Design review of the part built by this model. Coordinates are the model's own, in mm. A direction names the side the tool comes from. Coordinates: 2 decimals unless noted, no trailing zeros. Loops run counter-clockwise (first coordinate to the right, second up) from the corner with the lowest first, then second, coordinate; pieces in that order, holes last.
from build123d import *

# Parameters (mm, degrees)
SERVO_SHELF_START                        = -36.480025
SKETCH1_W                                = 48
SKETCH1_H                                = 38
SKETCH1_W_2                              = 13
SKETCH1_H_2                              = 24.35
SERVO_SHELF_DEPTH                        = 3
OUTBOARD_RISER_START                     = -34.480025
SKETCH2_W                                = 6
SKETCH2_H                                = 14
OUTBOARD_RISER_DEPTH                     = 33.480025
PLATE_ATTACHMENT_FOOT_START              = -2
SKETCH3_W                                = 20
SKETCH3_H                                = 14
PLATE_ATTACHMENT_FOOT_DEPTH              = 2
SKETCH4_R                                = 1.45
SERVO_PAD_D2P9_DEPTH                     = 2.01
SKETCH5_R                                = 2.6
SERVO_PAD_CSK_D5P2_90DEG_DEPTH           = 1.15
SERVO_PAD_CSK_D5P2_90DEG_DRAFT           = -45
SERVO_PAD_CSK_D5P2_90DEG_PROFILE_2_DEPTH = 1.15
SERVO_PAD_CSK_D5P2_90DEG_PROFILE_2_DRAFT = -45
SERVO_EAR_SUPPORTS_H2P2_START            = -33.480025
SKETCH6_R                                = 2.5
SERVO_EAR_SUPPORTS_H2P2_DEPTH            = 2.2
SKETCH7_R                                = 1.2
SERVO_EAR_D2P4_THROUGH_DEPTH             = 5.21


with BuildPart() as part:
    # Sketch1 → Servo_Shelf (new body)
    with BuildSketch(Plane.XY.offset(SERVO_SHELF_START)):
        with Locations((-46, 19)):
            Rectangle(SKETCH1_W, SKETCH1_H)
        with Locations((-60, 18.825)):
            Rectangle(SKETCH1_W_2, SKETCH1_H_2, mode=Mode.SUBTRACT)
    extrude(amount=SERVO_SHELF_DEPTH)

    # Sketch2 → Outboard_Riser (add)
    with BuildSketch(Plane.XY.offset(OUTBOARD_RISER_START)):
        with Locations((-37, 21)):
            Rectangle(SKETCH2_W, SKETCH2_H)
    extrude(amount=OUTBOARD_RISER_DEPTH)

    # Sketch3 → Plate_Attachment_Foot (add)
    with BuildSketch(Plane.XY.offset(PLATE_ATTACHMENT_FOOT_START)):
        with Locations((-30, 21)):
            Rectangle(SKETCH3_W, SKETCH3_H)
    extrude(amount=PLATE_ATTACHMENT_FOOT_DEPTH)

    # Sketch4 → Servo_Pad_D2p9 (cut)
    with BuildSketch(Plane(origin=(0, 0, -2), x_dir=(-1, 0, 0), z_dir=(0, 0, -1))):
        with Locations((25, 18)):
            Circle(SKETCH4_R)
        with Locations((25, 25)):
            Circle(SKETCH4_R)
    extrude(amount=-SERVO_PAD_D2P9_DEPTH, mode=Mode.SUBTRACT)


with BuildPart() as servo_pad_csk_d5p2_90deg_tool:
    # Sketch5 → Servo_Pad_CSK_D5p2_90deg (with draft: the straight prism first)
    with BuildSketch(Plane(origin=(0, 0, -2), x_dir=(-1, 0, 0), z_dir=(0, 0, -1))):
        with Locations((25, 18)):
            Circle(SKETCH5_R)
    extrude(amount=-SERVO_PAD_CSK_D5P2_90DEG_DEPTH)
    # Servo_Pad_CSK_D5p2_90deg: the draft: its side faces are tilted about the plane it starts from
    servo_pad_csk_d5p2_90deg_sides = [servo_pad_csk_d5p2_90deg_tool.faces().sort_by_distance(p)[0] for p in [
        (-22.4, 18, -1.425),
    ]]
    draft(servo_pad_csk_d5p2_90deg_sides, Plane(origin=(0, 0, -2), x_dir=(-1, 0, 0), z_dir=(0, 0, -1)), SERVO_PAD_CSK_D5P2_90DEG_DRAFT)


with BuildPart() as part_1:
    add(part.part)

    # Servo_Pad_CSK_D5p2_90deg: cut by servo_pad_csk_d5p2_90deg_tool
    add(servo_pad_csk_d5p2_90deg_tool.part, mode=Mode.SUBTRACT)


with BuildPart() as servo_pad_csk_d5p2_90deg_profile_2_tool:
    # Sketch5 → Servo_Pad_CSK_D5p2_90deg profile 2 (with draft: the straight prism first)
    with BuildSketch(Plane(origin=(0, 0, -2), x_dir=(-1, 0, 0), z_dir=(0, 0, -1))):
        with Locations((25, 25)):
            Circle(SKETCH5_R)
    extrude(amount=-SERVO_PAD_CSK_D5P2_90DEG_PROFILE_2_DEPTH)
    # Servo_Pad_CSK_D5p2_90deg profile 2: the draft: its side faces are tilted about the plane it starts from
    servo_pad_csk_d5p2_90deg_profile_2_sides = [servo_pad_csk_d5p2_90deg_profile_2_tool.faces().sort_by_distance(p)[0] for p in [
        (-22.4, 25, -1.425),
    ]]
    draft(servo_pad_csk_d5p2_90deg_profile_2_sides, Plane(origin=(0, 0, -2), x_dir=(-1, 0, 0), z_dir=(0, 0, -1)), SERVO_PAD_CSK_D5P2_90DEG_PROFILE_2_DRAFT)


with BuildPart() as part_2:
    add(part_1.part)

    # Servo_Pad_CSK_D5p2_90deg profile 2: cut by servo_pad_csk_d5p2_90deg_profile_2_tool
    add(servo_pad_csk_d5p2_90deg_profile_2_tool.part, mode=Mode.SUBTRACT)

    # Sketch6 → Servo_Ear_Supports_H2p2 (add)
    with BuildSketch(Plane.XY.offset(SERVO_EAR_SUPPORTS_H2P2_START)):
        with Locations(Location((-60, 4.55, 0), (0, 0, 122.859880379))):
            Circle(SKETCH6_R)
        with Locations(Location((-60, 32.75, 0), (0, 0, 224.427004001))):
            Circle(SKETCH6_R)
    extrude(amount=SERVO_EAR_SUPPORTS_H2P2_DEPTH)

    # Sketch7 → Servo_Ear_D2p4_Through (cut)
    with BuildSketch(Plane.XY.offset(-31.280025)):
        with Locations((-60, 4.55)):
            Circle(SKETCH7_R)
        with Locations((-60, 32.75)):
            Circle(SKETCH7_R)
    extrude(amount=-SERVO_EAR_D2P4_THROUGH_DEPTH, mode=Mode.SUBTRACT)


solid = part_2.part
Q1. Machinability: for faces 4 (the flat face through (-27, 21, -2)), 5 (the cylindrical face through (-57.646, 3.709, -32.395)), 6 (the flat face through (-35, 28, -14)), 7 (the flat face through (-22, 19, -35)), which of the approach directions +Z, -Z, +X, -X, +Y, -Y give a long, thin tool a straight path to every point of the face, cutting with its end or side? Answer none if there is none.
Q2. Take a section at B-B, the plane y = 10.5. Write out the cut boundary in (x, z).
Q3. Take a section at C-C, the plane x = -31.5. Write out the cut boundary in (y, z).
Q4. Clearance check with flat-ended pins moving along their axes: pin 1 Ø5 at (y, z) = (27.5, -22.5) entering from -X; pin 2 Ø3 at (x, y) = (-60, 32.75) entering from +Z; pin 3 Ø2.5 at (y, z) = (16.5, -34.5) entering from +X. State where each tip first meets the part, or that it passes through.
Q5. Take a section at A-A, the plane x = -25. Write out the cut boundary in (y, z).
Q6. For line 1 (Y direction, x = -60, z = -35.25); line 2 (Y direction, x = -25, z = -0.45); line 3 (X direction, y = 17, z = -8), list the stretches that pass through material, from the lowest coordinate up.
Q7. Take a section at D-D, the plane y = 18. Write out the cut boundary in (x, z), then the cut area to 3 significant figures.
Q8. The part is to be moulded in two halves that separate along Y. For faces 1 (the cylindrical face through (-26.339, 17.445, -0.431)), 2 (the flat face through (-30, 21, 0)), 3 (the flat face through (-35, 14, -14)), say which applies: pulls with the +Y half, pulls with the -Y half, needs draft (parallel to the pull), parting line crosses it, or undercut.
Entries:
1. face 4: +X, +Y, -Y
1. face 5: +Z
1. face 6: +Z, +X, -X, +Y
1. face 7: -Z, +X, +Y, -Y
2. outline: (-70, -36.48) - (-66.5, -36.48) - (-66.5, -33.48) - (-70, -33.48) - close; (-53.5, -36.48) - (-22, -36.48) - (-22, -33.48) - (-53.5, -33.48) - close
3. outline: (0, -36.48) - (38, -36.48) - (38, -33.48) - (0, -33.48) - close; (14, -2) - (28, -2) - (28, 0) - (14, 0) - close
4. pin 1: stops at x = -40
4. pin 2: stops at z = -31.28
4. pin 3: stops at x = -22
5. outline: (0, -36.48) - (38, -36.48) - (38, -33.48) - (0, -33.48) - close; (14, -2) - (15.4, -2) - (16.55, -0.85) - (16.55, 0) - (14, 0) - close; (19.45, -0.85) - (20.6, -2) - (22.4, -2) - (23.55, -0.85) - (23.55, 0) - (19.45, 0) - close; (26.45, -0.85) - (27.6, -2) - (28, -2) - (28, 0) - (26.45, 0) - close
6. line 1: y = 0 to 3.35, 5.75 to 6.65, 31 to 31.55, 33.95 to 38
6. line 2: y = 14 to 16.55, 19.45 to 23.55, 26.45 to 28
6. line 3: x = -40 to -34
7. outline: (-70, -36.48) - (-66.5, -36.48) - (-66.5, -33.48) - (-70, -33.48) - close; (-53.5, -36.48) - (-22, -36.48) - (-22, -33.48) - (-34, -33.48) - (-34, -2) - (-27.6, -2) - (-26.45, -0.85) - (-26.45, 0) - (-40, 0) - (-40, -33.48) - (-53.5, -33.48) - close; (-23.55, -0.85) - (-22.4, -2) - (-20, -2) - (-20, 0) - (-23.55, 0) - close
7. area: 327 mm2
8. face 1: undercut
8. face 2: needs draft
8. face 3: pulls with the -Y half
